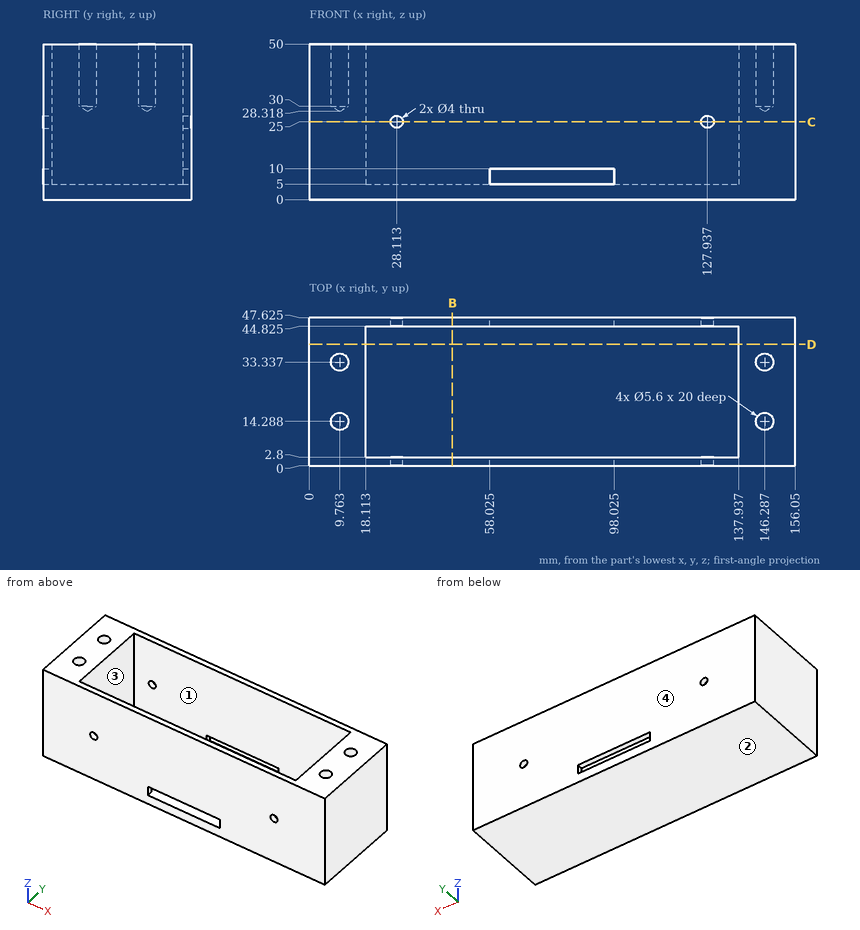
Could you check a few things on this drawing? It's one solid part, dimensions in mm from its lowest x, y, z. Coordinates: 2 decimals unless noted, no trailing zeros. Loops run counter-clockwise (first coordinate to the right, second up) from the corner with the lowest first, then second, coordinate; pieces in that order, holes last. Notation, with made-up numbers: (87, 88.5) - (104, 88.5) arc R38 ccw to (104, 127.5) - close; hole circle Ø10 at (-33, -14.5). An arc over 180 degrees is marked (long way). Answer as a JSON object with one key per item and string values. Group by question number.
Item 1: If we section it at C-C (z = 25): State how many separate pieces and enclosed holes the cut face has, plus the area to 3 significant figures.
Item 2: If we section it at D-D (y = 39): List the corners of the cut face in (x, z) for me, plus the area to 3 significant figures.
Item 3: If we mould it in two halves opening along Y, with no side actions, what happens to the marked faces 1, 2, 3 and 4? For each: released by +Y, released by -Y, zero draft, split by the parting line, or undercut.
Item 4: If we section it at B-B (x = 46): List the corners of the cut face in (y, z) for me (1 decimal).
Item 5: For pin 1 (12 mm diameter, centred on x = 135.5, y = 23.5, fed in from +Z); pin 2 (4 mm diameter, centred on x = 135, y = 14, fed in from +Z); pin 3 (3.5 mm diameter, centred on x = 127.937, z = 25, fed in from +Y), each with a flat end and sliding along its axis, tell me the tip position at first contact or that it passes through.
Item 6: If I drill on L1, parallel to X at y = 20, z = 45.5; L2, parallel to Y at x = 95, z = 13 (1 decimal); L3, parallel to X at y = 32, z = 35.5, over which ranges is the centre line in solid material (lowest first)? Write a range as from..to.
Returned:
{
 "1": {"separate pieces": "4", "enclosed holes": "0", "area": "2,350 mm²"},
 "2": {"outline": "(0, 0) - (156.05, 0) - (156.05, 50) - (137.94, 50) - (137.94, 5) - (18.11, 5) - (18.11, 50) - (0, 50) - close", "area": "2,410 mm²"},
 "3": {"face 1": "undercut", "face 2": "zero draft", "face 3": "undercut", "face 4": "released by +Y"},
 "4": {"outline": "(0, 0) - (47.6, 0) - (47.6, 50) - (44.8, 50) - (44.8, 5) - (2.8, 5) - (2.8, 50) - (0, 50) - close"},
 "5": {"pin 1": "stops at z = 50", "pin 2": "stops at z = 5", "pin 3": "passes through"},
 "6": {"L1": "x = 0..18.11, 137.94..156.05", "L2": "y = 0..2.8, 44.8..47.6", "L3": "x = 0..7.3, 12.22..18.11, 137.94..143.83, 148.75..156.05"}
}
